Job drawing, mm, ordinate dimensions from the low corner. One solid piece. Coordinates: 2 decimals unless noted, no trailing zeros. Loops run counter-clockwise (first coordinate to the right, second up) from the corner with the lowest first, then second, coordinate; pieces in that order, holes last. Notation, with made-up numbers: (1.5, 21) - (22.5, 21) arc R9 ccw to (22.5, 25) - close; hole circle Ø8 at (57, 21). An arc over 180 degrees is marked (long way). Use a Markdown table: item, result. Add a question column.
1) Pull direction Z, two halves, no side cores. Call the marked faces 1, 2 and 3: +Z half, -Z half, draft (parallel to the pull), parting line (faces both ways), or undercut.
2) Band-saw the part on C-C (x = 7.75). Give the cut face in (y, z).
3) Probe probe 1 along Y at (x, z) = (4, 34.5); probe 2 along Y at (x, z) = (5, 12) (1 decimal); probe 3 along Z at (x, y) = (8, 30). List the from-to ranges inside material, lowest first. Write a range as [from, to].
4) Band-saw the part on A-A (y = 26). Give the cut face in (x, z).
5) Drop flat-ended pins along their axis: P1, Ø10, axis at y = 9, z = 13.5, coming from the -X side; P2, Ø1.5, axis at x = 1, y = 35, coming from the -Z side; P3, Ø3, axis at x = 6.5, z = 33.5, coming from the -Y side; P4, Ø1.5, axis at x = 9, z = 41, coming from the -Y side. Give the stop position or say it passes through.
6) Band-saw the part on B-B (x = 3.25). Give the cut face in (y, z).
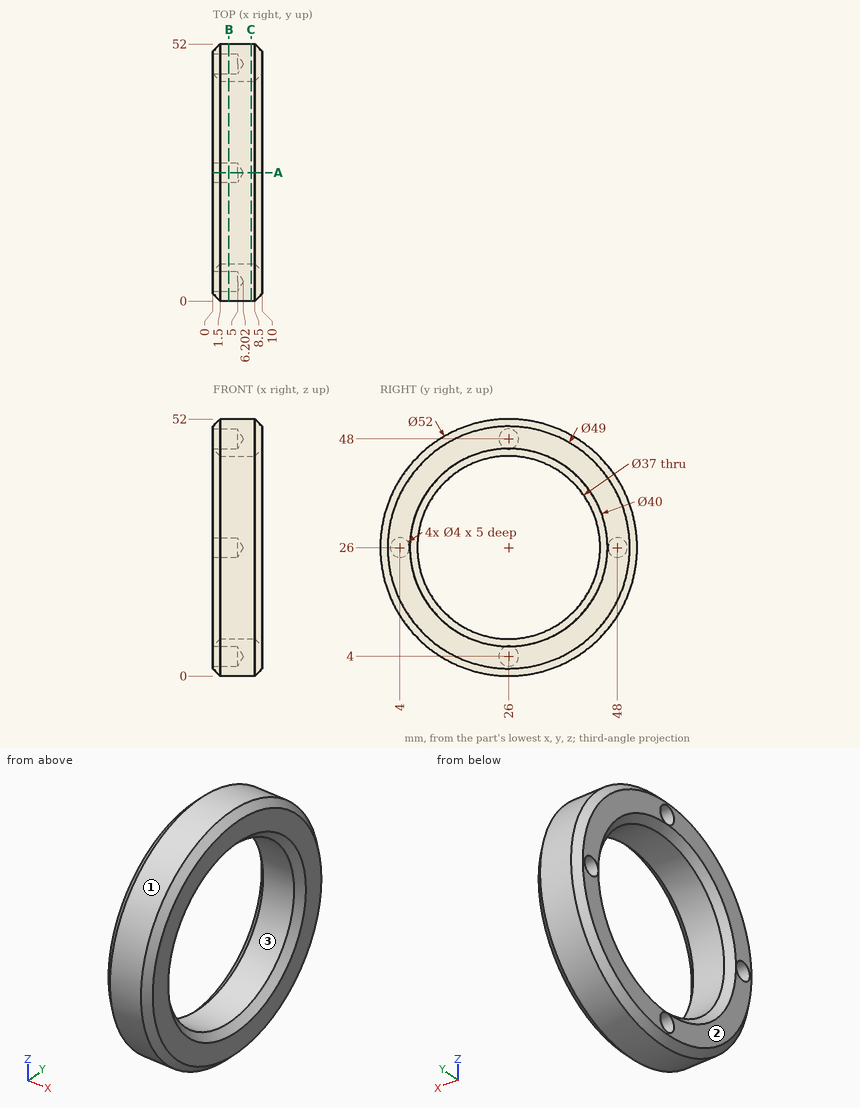
Answer block:
| question | item | result |
|---|---|---|
| 1 | face 1 | parting line |
| 1 | face 2 | draft |
| 1 | face 3 | undercut |
| 2 | outline | circle Ø52 at (26, 26); hole circle Ø37 at (26, 26) |
| 3 | probe 1 | [1.43, 9.57], [42.43, 50.57] |
| 3 | probe 2 | [4.1, 13.9], [38.1, 47.9] |
| 3 | probe 3 | [0.31, 7.94], [44.06, 51.69] |
| 4 | outline | (0, 1.5) - (1.5, 0) - (8.5, 0) - (10, 1.5) - (10, 6) - (8.5, 7.5) - (1.5, 7.5) - (0, 6) - (5, 6) - (6.2, 4) - (5, 2) - (0, 2) - close; (0, 46) - (1.5, 44.5) - (8.5, 44.5) - (10, 46) - (10, 50.5) - (8.5, 52) - (1.5, 52) - (0, 50.5) - (0, 50) - (5, 50) - (6.2, 48) - (5, 46) - close |
| 5 | P1 | x = 0 |
| 5 | P2 | z = 1.41 |
| 5 | P3 | y = 0.7 |
| 5 | P4 | y = 4.38 |
| 6 | outline | circle Ø52 at (26, 26); hole circle Ø4 at (4, 26); hole circle Ø37 at (26, 26); hole circle Ø4 at (26, 4); hole circle Ø4 at (26, 48); hole circle Ø4 at (48, 26) |
